```python
from build123d import *

# Parameters (mm, degrees)
F0_R     = 3.175
F0_R_2   = 2.4892
F0_R_3   = 9.525
F1_DEPTH = 12.7
F2_R     = 5.08


with BuildPart() as f1:
    # F0 (on Front) → F1 (new body)
    with BuildSketch(Plane.XZ):
        with BuildLine():
            Line((-31.75, -25.4), (31.75, -25.4))
            Line((31.75, -25.4), (31.75, 38.1))
            ThreePointArc((31.75, 38.1), (28.0302561211, 47.0802561211), (19.05, 50.8))
            Line((19.05, 50.8), (-19.05, 50.8))
            ThreePointArc((-19.05, 50.8), (-28.0302561211, 47.0802561211), (-31.75, 38.1))
            Line((-31.75, 38.1), (-31.75, -25.4))
        make_face()
        with Locations((-19.05, -12.7)):
            Circle(F0_R, mode=Mode.SUBTRACT)
        with Locations((-17.7292, 7.6708)):
            Circle(F0_R_2, mode=Mode.SUBTRACT)
        with Locations((19.05, -12.7)):
            Circle(F0_R, mode=Mode.SUBTRACT)
        with Locations((0, 25.4)):
            Circle(F0_R_3, mode=Mode.SUBTRACT)
        with Locations((17.7292, 43.1292)):
            Circle(F0_R_2, mode=Mode.SUBTRACT)
    extrude(amount=F1_DEPTH)

    # F2
    f2_edges = [f1.edges().sort_by_distance(p)[0] for p in [
        (31.75, -6.35, -25.4),
        (-31.75, -6.35, -25.4),
    ]]
    fillet(f2_edges, radius=F2_R)


solid = f1.part
```
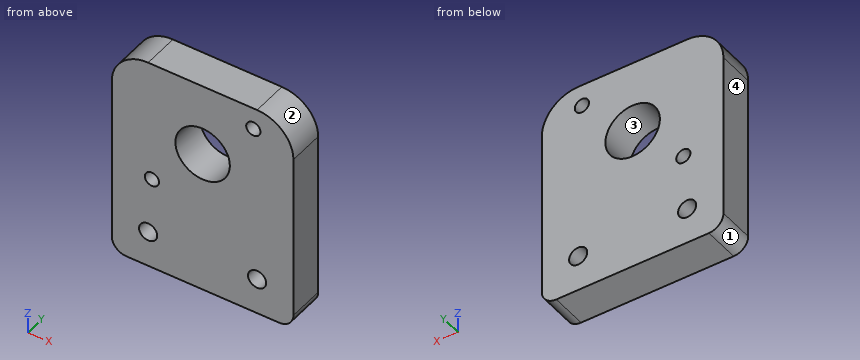
Work out the finished part from the listing and answer in its coordinate system (mm). Face numbers are marked on the shaded views. Round coordinates to 2 decimals unless told otherwise and drop trailing zeros. Write each loop counter-clockwise with the first axis right and the second up, starting at its lowest first coordinate (ties: lowest second). Pieces come first, ordered by that corner, then holes. Notation, with made-up numbers: (21.25, 54.5) -> (80.25, 54.5) arc R24 ccw to (80.25, 93.5) -> close; hole circle Ø6 at (-18.5, -17.5). An arc over 180 degrees is marked (long way). Write each question's results on one line, items separated by ' | '.
Q1. Flat-ended cylindrical pins translate along their axes: P1, Ø6, axis at y = -7, z = 42, coming from the +X side; P2, Ø2, axis at x = -24, z = 31.5, coming from the +Y side. Find the tip coordinate at first contact, or state that the pin passes through.
Data:
P1: x = 31.72 | P2: y = 0
Q2. Section A-A, the plane z = 25.4 is taken. Write down the section's boundary in (x, y) (3 decimals).
Data:
outline: (-31.75, -12.7) -> (-9.525, -12.7) -> (-9.525, 0) -> (-31.75, 0) -> close; (9.525, -12.7) -> (31.75, -12.7) -> (31.75, 0) -> (9.525, 0) -> close
Q3. Section B-B, the plane x = 0 is taken. Write down the section's boundary in (y, z) (3 decimals).
Data:
outline: (-12.7, -25.4) -> (0, -25.4) -> (0, 15.875) -> (-12.7, 15.875) -> close; (-12.7, 34.925) -> (0, 34.925) -> (0, 50.8) -> (-12.7, 50.8) -> close
Q4. Determine the mould class of the marked faces 1, 2, 3 and 4 for opening direction Z: released by +Z, released by -Z, zero draft, split by the parting line, or undercut.
Data:
face 1: released by -Z | face 2: released by +Z | face 3: undercut | face 4: zero draft
Q5. Straight lines are drawn through the part: line 1 along Z through (x, y) = (18, -6.75); line 2 along X through (y, z) = (-2.75, 26); line 3 along Z through (x, y) = (-19.05, -5) (3 decimals). For each, find the intervals that lie inside material, in ascending order. Write a range as [from, to].
Data:
line 1: [-25.4, -15.7], [-9.7, 40.65], [45.6, 50.8] | line 2: [-31.75, -9.51], [9.51, 31.75] | line 3: [-25.4, -15.875], [-9.525, 5.561], [9.781, 50.8]
Q6. Section D-D, the plane y = -9 is taken. Write down the section's boundary in (x, z) (3 decimals), then the cut area to 3 significant figures.
Data:
outline: (-31.75, -20.32) arc R5.08 ccw to (-26.67, -25.4) -> (26.67, -25.4) arc R5.08 ccw to (31.75, -20.32) -> (31.75, 38.1) arc R12.7 ccw to (19.05, 50.8) -> (-19.05, 50.8) arc R12.7 ccw to (-31.75, 38.1) -> close; hole circle Ø6.35 at (-19.05, -12.7); hole circle Ø4.978 at (-17.729, 7.671); hole circle Ø19.05 at (0, 25.4); hole circle Ø4.978 at (17.729, 43.129); hole circle Ø6.35 at (19.05, -12.7) | area: 4,370 mm^2
Q7. Section C-C, the plane z = -12.7 is taken. Write down the section's boundary in (x, y) (3 decimals).
Data:
outline: (-31.75, -12.7) -> (-22.225, -12.7) -> (-22.225, 0) -> (-31.75, 0) -> close; (-15.875, -12.7) -> (15.875, -12.7) -> (15.875, 0) -> (-15.875, 0) -> close; (22.225, -12.7) -> (31.75, -12.7) -> (31.75, 0) -> (22.225, 0) -> close
